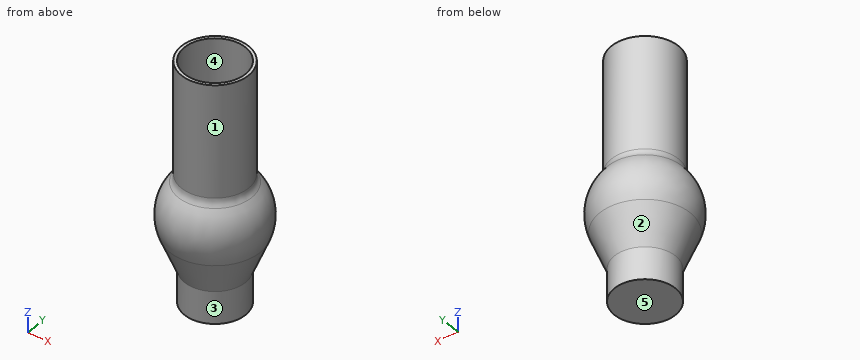
from build123d import *


with BuildPart() as f1:
    # F0 (on Front) → F1 (revolve)
    with BuildSketch(Plane.XZ):
        with BuildLine():
            ThreePointArc((22.5, 19.843135), (29.571752, 5.05089), (27.810744, -11.25))
            Line((27.810744, -11.25), (13.905372, -45.625))
            ThreePointArc((13.905372, -45.625), (8.385255, -52.437343), (0, -55))
            Line((0, -55), (0, -57))
            Line((0, -57), (20, -57))
            Line((20, -57), (20, -35.89201))
            Line((20, -35.89201), (29.664794, -12))
            ThreePointArc((29.664794, -12), (31.543202, 5.387616), (24, 21.16601))
            ThreePointArc((24, 21.16601), (22.516685, 23.629086), (22, 26.457513))
            Line((22, 26.457513), (22, 100))
            Line((22, 100), (20, 100))
            Line((20, 100), (20, 26.457513))
            ThreePointArc((20, 26.457513), (20.645857, 22.921979), (22.5, 19.843135))
        make_face()
    revolve(axis=Axis((0, 0, 55.570815), (0, 0, 1)))


solid = f1.part
Could you check a few things on this model? Use its own coordinates, in mm. Face numbers are marked on the shaded views. A direction names the side the tool comes from. Coordinates: 2 decimals unless noted, no trailing zeros. Loops run counter-clockwise (first coordinate to the right, second up) from the corner with the lowest first, then second, coordinate; pieces in that order, holes last.
1. For P1, Ø10, axis at y = -2.5, z = 37.5, coming from the -X side; P2, Ø1, axis at y = 18.5, z = 58, coming from the +X side; P3, Ø1.5, axis at x = -1.5, y = -21, coming from the -Z side, each with a flat end and sliding along its axis, tell me the tip position at first contact or that it passes through.
2. Imagine slicing it at A-A (z = 45). Please give me the cut outline in (x, y).
3. For the marked faces 1 and 2, which set-ups out of +Z, -Z, +X, -X, +Y, -Y let a thin tool reach every point of the face, with its end or its side?
4. We'd pull the mould along Y, two halves only. Please class the marked faces 3, 4 and 5: released by +Y, released by -Y, zero draft, split by the parting line, or undercut.
5. I need wall thicknesses on L1, parallel to Y at x = 0, z = 83; L2, parallel to X at y = 1, z = 46.5; L3, parallel to X at y = 14, z = 27.5. Which ranges of each line are inside material? Lowest first, please.
Computed values:
1. P1: stops at x = -22
1. P2: stops at x = 12.65
1. P3: stops at z = -35.14
2. outline: circle Ø44 at (0, 0); hole circle Ø40 at (0, 0)
3. face 1: +Z
3. face 2: -Z
4. face 3: split by the parting line
4. face 4: undercut
4. face 5: zero draft
5. L1: y = -22 to -20, 20 to 22
5. L2: x = -21.98 to -19.97, 19.97 to 21.98
5. L3: x = -16.97 to -14.28, 14.28 to 16.97
